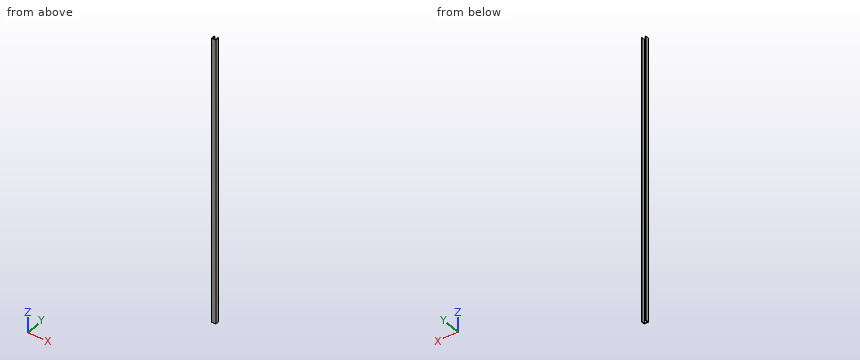
Autodesk Inventor part; units mm, degrees
ref_plane "YZ Plane" through (0, 0, 0) normal (1, 0, 0) x (0, 1, 0)
ref_plane "XZ Plane" through (0, 0, 0) normal (0, 1, 0) x (-1, 0, 0)
ref_plane "XY Plane" through (0, 0, 0) normal (0, 0, 1) x (1, 0, 0)
sketch "Sketch1" plane through (0, 0, 0) normal (0, 0, 1) x (1, 0, 0)
  line L0 (-6.6675, 0) -> (6.6675, 0)
  line L1 (0, -6.35) -> (0, 4.7625)
  line L2 (-3.175, 3.175) -> (-3.175, -3.175)
  line L3 (-3.175, -3.175) -> (3.175, -3.175)
  line L4 (3.175, -3.175) -> (3.175, 3.175)
  line L5 (4.7625, 3.175) -> (4.7625, -4.7625)
  line L6 (4.7625, -4.7625) -> (-4.7625, -4.7625)
  line L7 (-4.7625, -4.7625) -> (-4.7625, 3.175)
  line L8 (-3.175, 3.175) -> (-4.7625, 3.175)
  line L9 (3.175, 3.175) -> (4.7625, 3.175)
  point P0 (0, 0)
  point P1 (0, -3.175)
  point P2 (-3.175, 0)
  dimension "d0" = 1.5875
  dimension "d1" = 6.35
  dimension "d2" = 6.35
extrude "Extrusion1" add sketch "Sketch1" along normal mid plane 609.6 contours L7 L8 L2 L0 | L0 L2 L3 L1 L6 L7 | L1 L3 L4 L0 L5 L6 | L4 L9 L5 L0
properties part number "c-channel template" material "Aluminum-6061"
For this review, take the finished solid that the model builds, in its own axes (mm). Give positions to 0.01 mm unless a question says otherwise; leave off trailing zeros. Order: outer loops, then holes, each group sorted by start corner. A loop starts at its lowest first (then second) coordinate and runs counter-clockwise, first axis right, second up. Notation, with made-up numbers: (-23, 19) - (17, 19) arc R19 cw to (17, 37) - close; hole circle Ø5 at (-7.75, 24.5). An arc over 180 degrees is marked (long way). Answer as a JSON object with one key per item and string values. Group by question number.
Item 1: Wall thickness on line 1 along X through (y, z) = (2.75, 31) (1 decimal); line 2 along Y through (x, z) = (-1.75, 137) (1 decimal): over which ranges is each line inside the solid? List them lowest first.
Item 2: Clearance check with flat-ended pins moving along their axes: pin 1 Ø3 at (x, y) = (-2, -1) entering from +Z; pin 2 Ø5 at (x, z) = (-0.5, 18) entering from +Y (3 decimals). State where each tip first meets the part, or that it passes through.
Item 3: Take a section at A-A on y = 1.25. Give the boundary of the cut face in (x, z) (1 decimal).
Item 4: Take a section at C-C on x = 0.25. Give the boundary of the cut face in (y, z) (1 decimal), and give its area (3 significant figures).
Item 5: Take a section at B-B on z = 68. Give the boundary of the cut face in (x, y) (1 decimal), and give its area (3 significant figures).
Reported:
{
 "1": {"line 1": "-4.8 to -3.2, 3.2 to 4.8", "line 2": "-4.8 to -3.2"},
 "2": {"pin 1": "z = 304.8", "pin 2": "y = -3.175"},
 "3": {"outline": "(-4.8, -304.8) - (-3.2, -304.8) - (-3.2, 304.8) - (-4.8, 304.8) - close; (3.2, -304.8) - (4.8, -304.8) - (4.8, 304.8) - (3.2, 304.8) - close"},
 "4": {"outline": "(-4.8, -304.8) - (-3.2, -304.8) - (-3.2, 304.8) - (-4.8, 304.8) - close", "area": "968 mm^2"},
 "5": {"outline": "(-4.8, -4.8) - (4.8, -4.8) - (4.8, 3.2) - (3.2, 3.2) - (3.2, -3.2) - (-3.2, -3.2) - (-3.2, 3.2) - (-4.8, 3.2) - close", "area": "35.3 mm^2"}
}
